For this review, take the finished solid that the model builds, in its own axes (mm). Round coordinates to 2 decimals unless told otherwise and drop trailing zeros. Order: outer loops, then holes, each group sorted by start corner. A loop starts at its lowest first (then second) coordinate and runs counter-clockwise, first axis right, second up. Notation, with made-up numbers: (35, -6) -> (44, -6) arc R17 cw to (44, 13) -> close; hole circle Ø5 at (-28.75, 87.5). An arc over 180 degrees is marked (long way). Put each result on its own line as item: value. Start each with the question number.
```python
from build123d import *

# Parameters (mm, degrees)
SKETCH1_R             = 3
BOSS_EXTRUDE1_DEPTH   = 6.35
F_4_40_TAPPED_HOLE1_D = 2.2606
CHAMFER1_SIZE         = 2


with BuildPart() as part:
    # Sketch1 → Boss-Extrude1 (new body)
    with BuildSketch(Plane.XY):
        Polygon((-10, 0.807611845), (0.807611845, -10), (10, -10), (10, 10), (-10, 10), align=None)
        Circle(SKETCH1_R, mode=Mode.SUBTRACT)
    extrude(amount=BOSS_EXTRUDE1_DEPTH)

    # #4-40 Tapped Hole1 (through all)
    with Locations(Plane.XY.offset(6.35)):
        with Locations((-6.731, 6.731), (6.731, -6.731), (-6.731, -6.731), (6.731, 6.731)):
            Hole(F_4_40_TAPPED_HOLE1_D / 2)

    # Chamfer1
    chamfer1_edges = [part.edges().sort_by_distance(p)[0] for p in [
        (-10, 10, 3.175),
        (10, 10, 3.175),
        (10, -10, 3.175),
    ]]
    chamfer(chamfer1_edges, length=CHAMFER1_SIZE)


solid = part.part
```
Item 1: For L1, parallel to Y at x = 7.25, z = 1; L2, parallel to Y at x = 7, z = 3; L3, parallel to Y at x = 0, z = 3.5, list the stretches that pass through material, from the lowest coordinate up.
Item 2: Consider section A-A, the plane y = -7. Write out the cut boundary in (x, z).
Item 3: Consider section D-D, the plane x = -8.75. Write out the cut boundary in (y, z).
Item 4: Mouldability with a two-part tool opening along Y and no side actions: class faces 1 (the face through (5.687, 6.298, 3.131)), 2 (the face through (0, 10, 3)), 3 (the face through (-10, 4, 3)), 4 (the face through (4, -10, 3)) as +Y half, -Y half, draft (parallel to the pull), parting line (faces both ways), or undercut.
Item 5: Consider section B-B, the plane x = 2. Write out the cut boundary in (y, z), plus the area to 3 significant figures.
Item 6: Consider section C-C, the plane z = 3.75. Write out the cut boundary in (x, y).
Evaluation:
1. L1: y = -10 to -7.74, -5.73 to 5.73, 7.74 to 10
1. L2: y = -10 to -7.83, -5.63 to 5.63, 7.83 to 10
1. L3: y = -9.19 to -3, 3 to 10
2. outline: (-2.19, 0) -> (5.63, 0) -> (5.63, 6.35) -> (-2.19, 6.35) -> close; (7.83, 0) -> (10, 0) -> (10, 6.35) -> (7.83, 6.35) -> close
3. outline: (-0.44, 0) -> (9.25, 0) -> (9.25, 6.35) -> (-0.44, 6.35) -> close
4. face 1: undercut
4. face 2: +Y half
4. face 3: draft
4. face 4: -Y half
5. outline: (-10, 0) -> (-2.24, 0) -> (-2.24, 6.35) -> (-10, 6.35) -> close; (2.24, 0) -> (10, 0) -> (10, 6.35) -> (2.24, 6.35) -> close
5. area: 98.6 mm^2
6. outline: (-10, 0.81) -> (0.81, -10) -> (8, -10) -> (10, -8) -> (10, 8) -> (8, 10) -> (-8, 10) -> (-10, 8) -> close; hole circle Ø2.26 at (-6.73, 6.73); hole circle Ø6 at (0, 0); hole circle Ø2.26 at (6.73, -6.73); hole circle Ø2.26 at (6.73, 6.73)
